from build123d import *

# Parameters (mm, degrees)
SKETCH_1_W          = 125
SKETCH_1_H          = 78
SKETCH_1_R          = 3.6
SKETCH_1_R_2        = 1.6
SKETCH_1_W_2        = 120
SKETCH_1_H_2        = 74
EXTRUDE_1_DEPTH     = 13
SHELL_1_T           = -2
SKETCH_3_R          = 2.5
SKETCH_3_R_2        = 1.6
EXTRUDE_2_DEPTH     = 5
CUT_EXTRUDE_1_DEPTH = 5
FILLET_1_R          = 5
FILLET_2_R          = 2


with BuildPart() as part:
    # 草图1 → 凸台-拉伸1 (new body)
    # profile 1 of 6: a face of its own
    with BuildSketch(Plane.XY):
        Rectangle(SKETCH_1_W, SKETCH_1_H)
        with Locations((-57, -33.5)):
            Circle(SKETCH_1_R, mode=Mode.SUBTRACT)
        with Locations((-57, 33.5)):
            Circle(SKETCH_1_R, mode=Mode.SUBTRACT)
        with Locations((57, -33.5)):
            Circle(SKETCH_1_R, mode=Mode.SUBTRACT)
        with Locations((57, 33.5)):
            Circle(SKETCH_1_R, mode=Mode.SUBTRACT)
    # profile 2 of 6: a face of its own
    with BuildSketch(Plane.XY):
        with Locations((57, 33.5)):
            Circle(SKETCH_1_R)
        with Locations((57, 33.5)):
            Circle(SKETCH_1_R_2, mode=Mode.SUBTRACT)
    # profile 3 of 6: a face of its own
    with BuildSketch(Plane.XY):
        with Locations((-57, -33.5)):
            Circle(SKETCH_1_R)
        with Locations((-57, -33.5)):
            Circle(SKETCH_1_R_2, mode=Mode.SUBTRACT)
    # profile 4 of 6: a face of its own
    with BuildSketch(Plane.XY):
        with Locations((57, -33.5)):
            Circle(SKETCH_1_R)
        with Locations((57, -33.5)):
            Circle(SKETCH_1_R_2, mode=Mode.SUBTRACT)
    # profile 5 of 6: a face of its own
    with BuildSketch(Plane.XY):
        with Locations((-57, 33.5)):
            Circle(SKETCH_1_R)
        with Locations((-57, 33.5)):
            Circle(SKETCH_1_R_2, mode=Mode.SUBTRACT)
    # profile 6 of 6: a face of its own
    with BuildSketch(Plane.XY):
        Rectangle(SKETCH_1_W_2, SKETCH_1_H_2)
    extrude(amount=EXTRUDE_1_DEPTH)

    # 抽壳1
    shell_1_openings = [part.faces().sort_by_distance(p)[0] for p in [
        (0, 0, 13),
    ]]
    offset(amount=SHELL_1_T, openings=shell_1_openings, kind=Kind.INTERSECTION)

    # 草图3 → 凸台-拉伸2 (add)
    # profile 1 of 4: a face of its own
    with BuildSketch(Plane.XY.offset(2)):
        with Locations((-56.5, 33.5)):
            Circle(SKETCH_3_R)
        with Locations((-56.5, 33.5)):
            Circle(SKETCH_3_R_2, mode=Mode.SUBTRACT)
    # profile 2 of 4: a face of its own
    with BuildSketch(Plane.XY.offset(2)):
        with Locations(Location((56.5, 33.5, 0), (0, 0, 180))):
            Circle(SKETCH_3_R)
        with Locations(Location((56.5, 33.5, 0), (0, 0, 180))):
            Circle(SKETCH_3_R_2, mode=Mode.SUBTRACT)
    # profile 3 of 4: a face of its own
    with BuildSketch(Plane.XY.offset(2)):
        with Locations((56.5, -33.5)):
            Circle(SKETCH_3_R)
        with Locations((56.5, -33.5)):
            Circle(SKETCH_3_R_2, mode=Mode.SUBTRACT)
    # profile 4 of 4: a face of its own
    with BuildSketch(Plane.XY.offset(2)):
        with Locations(Location((-56.5, -33.5, 0), (0, 0, 180))):
            Circle(SKETCH_3_R)
        with Locations(Location((-56.5, -33.5, 0), (0, 0, 180))):
            Circle(SKETCH_3_R_2, mode=Mode.SUBTRACT)
    extrude(amount=EXTRUDE_2_DEPTH)

    # 草图5 → 切除-拉伸1 (cut)
    with BuildSketch(Plane.ZY.offset(62.5)):
        Polygon((2.138422059, 12.60316827), (10.861577941, 12.60316827), (10.861577941, -12.60316827), (2.138422059, -12.60316827), (0, -12.60316827), (0, 12.60316827), align=None)
    extrude(amount=-CUT_EXTRUDE_1_DEPTH, mode=Mode.SUBTRACT)

    # 圆角1
    fillet_1_edges = [part.edges().sort_by_distance(p)[0] for p in [
        (62.5, -39, 6.5),
        (-62.5, -39, 6.5),
        (-62.5, 39, 6.5),
        (62.5, 39, 6.5),
    ]]
    fillet(fillet_1_edges, radius=FILLET_1_R)

    # 圆角2
    fillet_2_edges = [part.edges().sort_by_distance(p)[0] for p in [
        (-60.5, 37, 7.5),
        (60.5, 37, 7.5),
        (60.5, -37, 7.5),
        (-60.5, -37, 7.5),
    ]]
    fillet(fillet_2_edges, radius=FILLET_2_R)


solid = part.part
The listing builds one solid part. Answer for the finished solid, in the listing's coordinates (mm). A direction names the side the tool comes from. Round coordinates to 2 decimals unless told otherwise and drop trailing zeros. Order: outer loops, then holes, each group sorted by start corner. A loop starts at its lowest first (then second) coordinate and runs counter-clockwise, first axis right, second up. Notation, with made-up numbers: (85, -1.75) -> (97, -1.75) arc R32 cw to (97, 28.25) -> close; hole circle Ø11 at (8.25, 74.5). An arc over 180 degrees is marked (long way). Put each result on its own line as item: value.
Q1. Section C-C, the plane y = 9 is taken. Write down the section's boundary in (x, z), and give its area (3 significant figures).
Results list:
outline: (-62.5, 10.86) -> (-60.5, 10.86) -> (-60.5, 13) -> (-62.5, 13) -> close; (-57.5, 0) -> (62.5, 0) -> (62.5, 13) -> (60.5, 13) -> (60.5, 2) -> (-57.5, 2) -> close
area: 266 mm^2
Q2. Section B-B, the plane x = -25.5 is taken. Write down the section's boundary in (y, z).
Results list:
outline: (-39, 0) -> (39, 0) -> (39, 13) -> (37, 13) -> (37, 2) -> (-37, 2) -> (-37, 13) -> (-39, 13) -> close
Q3. Each of these flat-tipped pins is pushed along its axis until it touches: P1, Ø10, axis at x = 32, y = 7, coming from the +Z side; P2, Ø0.6, axis at y = -1.5, z = 0.5, coming from the -X side; P3, Ø1.5, axis at x = 55.5, y = 34, coming from the +Z side; P4, Ø4, axis at x = -59.5, z = 7, coming from the -Y side. Where does it stop, or does it pass through?
Results list:
P1: z = 2
P2: x = -57.5
P3: z = 7
P4: y = -39
Q4. Which of the six approach directions +Z, -Z, +X, -X, +Y, -Y give full straight-line access (tool end or side, diameter ignored) to faces 1 (the flat face through (-61, 12.603, 4)), 2 (the flat face through (0, 38, 13)), 3 (the flat face through (-57, 34, 2))?
Results list:
face 1: -Z, -X
face 2: +Z, +X, -X, +Y, -Y
face 3: +Z
Q5. Section A-A, the plane z = 3.5 is taken. Count the separate pieces of the cut face and the enclosed holes in it, and give its area (3 significant figures).
Results list:
separate pieces: 5
enclosed holes: 4
area: 774 mm^2
Q6. Section D-D, the plane z = 8.75 is taken. Write down the section's boundary in (x, y).
Results list:
outline: (-62.5, -34) arc R5 ccw to (-57.5, -39) -> (57.5, -39) arc R5 ccw to (62.5, -34) -> (62.5, 34) arc R5 ccw to (57.5, 39) -> (-57.5, 39) arc R5 ccw to (-62.5, 34) -> (-62.5, 12.6) -> (-60.5, 12.6) -> (-60.5, 35) arc R2 cw to (-58.5, 37) -> (58.5, 37) arc R2 cw to (60.5, 35) -> (60.5, -35) arc R2 cw to (58.5, -37) -> (-58.5, -37) arc R2 cw to (-60.5, -35) -> (-60.5, -12.6) -> (-62.5, -12.6) -> close
Q7. Consider line 1 along Y through (x, z) = (-56.5, 4.65); line 2 along Y through (x, z) = (-6.5, 5.5); line 3 along X through (y, z) = (22, 9). Determine where each line is inside the solid, lowest interval first.
Results list:
line 1: -39 to -37, -36 to -35.1, -31.9 to -31, 31 to 31.9, 35.1 to 36, 37 to 39
line 2: -39 to -37, 37 to 39
line 3: -62.5 to -60.5, 60.5 to 62.5
Q8. Determine the mould class of faces 4 (the flat face through (62.5, 0, 6)), 5 (the cylindrical face through (57.24, -34.92, 4.46)), 6 (the flat face through (-1, 1, 0)) for opening direction X: pulls with the +X half, pulls with the -X half, needs draft (parallel to the pull), parting line crosses it, or undercut.
Results list:
face 4: pulls with the +X half
face 5: undercut
face 6: needs draft
